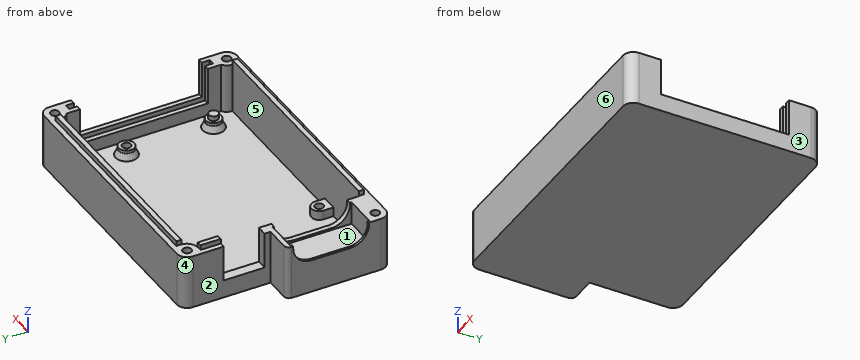
```python
from build123d import *

# Parameters (mm, degrees)
PAD_DEPTH       = 1.5
PAD001_DEPTH    = 15.9
SKETCH003_R     = 2.5
PAD002_DEPTH    = 3
SKETCH004_R     = 1.5
PAD003_DEPTH    = 1.6
SKETCH005_W     = 70.1
SKETCH005_H     = 1.6
SKETCH005_W_2   = 1.6
SKETCH005_H_2   = 11.9
SKETCH005_W_3   = 73.4
PAD004_DEPTH    = 1.6
SKETCH007_W     = 1.9
SKETCH007_H     = 46.1
POCKET001_DEPTH = 14.35
SKETCH008_W     = 5.6
SKETCH008_H     = 41.02
POCKET002_DEPTH = 11.81
SKETCH009_W     = 4.8
SKETCH009_H     = 13.1
POCKET003_DEPTH = 13.2
SKETCH010_R     = 1.4
POCKET004_DEPTH = 15.9
POCKET_DEPTH    = 6.7
SKETCH014_W     = 10.3
SKETCH014_H     = 25.3
POCKET006_DEPTH = 0.65
SKETCH023_R     = 1.4
POCKET014_DEPTH = 4
CHAMFER_SIZE2   = 2
CHAMFER_SIZE    = 1
FILLET_R        = 3.3
FILLET001_R     = 1.6
FILLET002_R     = 6


with BuildPart() as part:
    # Sketch → Pad (new body)
    with BuildSketch(Plane.XY):
        Polygon((13.3, 49.3), (13.3, 77.5), (96.8, 77.5), (96.8, 15.8), (3.9, 15.8), (3.9, 49.3), align=None)
    extrude(amount=PAD_DEPTH)

    # Sketch001 (on Face8 of Pad) → Pad001 (join)
    with BuildSketch(Plane.XY.offset(1.5)):
        Polygon((96.8, 77.5), (13.3, 77.5), (13.3, 49.3), (3.9, 49.3), (3.9, 15.8), (96.8, 15.8), align=None)
        with BuildLine():
            Line((16.6, 70.9), (16.6, 19.1))
            Line((16.6, 19.1), (90.2, 19.1))
            ThreePointArc((91.7, 21.865863), (90.599138, 20.673213), (90.2, 19.1))
            Line((91.7, 21.865863), (91.7, 71.434137))
            ThreePointArc((90.2, 74.2), (90.599138, 72.626787), (91.7, 71.434137))
            Line((90.2, 74.2), (19.9, 74.2))
            ThreePointArc((16.6, 70.9), (18.933452, 71.866548), (19.9, 74.2))
        make_face(mode=Mode.SUBTRACT)
    extrude(amount=PAD001_DEPTH)

    # Sketch003 (on Face9 of Pad001) → Pad002 (join)
    with BuildSketch(Plane.XY.offset(1.5)):
        with Locations((86, 55.35)):
            Circle(SKETCH003_R)
        with Locations((86, 27.45)):
            Circle(SKETCH003_R)
        with BuildLine():
            ThreePointArc((36.4, 22.35), (33.9, 24.85), (31.4, 22.35))
            Line((31.4, 22.35), (31.4, 18))
            Line((36.4, 18), (31.4, 18))
            Line((36.4, 22.35), (36.4, 18))
        make_face()
        with BuildLine():
            ThreePointArc((32.95, 70.55), (35.2, 68.3), (37.45, 70.55))
            Line((37.45, 70.55), (37.45, 75.55))
            Line((32.95, 75.55), (37.45, 75.55))
            Line((32.95, 70.55), (32.95, 75.55))
        make_face()
    extrude(amount=PAD002_DEPTH)

    # Sketch004 (on Face28 of Pad002) → Pad003 (join)
    with BuildSketch(Plane.XY.offset(4.5)):
        with Locations((35.2, 70.55)):
            Circle(SKETCH004_R)
        with Locations((86, 27.45)):
            Circle(SKETCH004_R)
    extrude(amount=PAD003_DEPTH)

    # Sketch005 (on Face1 of Pad003) → Pad004 (join)
    with BuildSketch(Plane.XY.offset(17.4)):
        with Locations((55.05, 75)):
            Rectangle(SKETCH005_W, SKETCH005_H)
        with Locations((15.8, 64.85)):
            Rectangle(SKETCH005_W_2, SKETCH005_H_2)
        with Locations((53.4, 18.3)):
            Rectangle(SKETCH005_W_3, SKETCH005_H)
    extrude(amount=PAD004_DEPTH)

    # Sketch007 (on Face1 of Pad004) → Pocket001 (cut)
    with BuildSketch(Plane.XY.offset(17.4)):
        with Locations((94.25, 46.65)):
            Rectangle(SKETCH007_W, SKETCH007_H)
    extrude(amount=-POCKET001_DEPTH, mode=Mode.SUBTRACT)

    # Sketch008 (on Face1 of Pocket001) → Pocket002 (cut)
    with BuildSketch(Plane.XY.offset(17.4)):
        with Locations((94.25, 46.65)):
            Rectangle(SKETCH008_W, SKETCH008_H)
    extrude(amount=-POCKET002_DEPTH, mode=Mode.SUBTRACT)

    # Sketch009 (on Face41 of Pocket002) → Pocket003 (cut)
    with BuildSketch(Plane.XY.offset(19)):
        with Locations((14.6, 57.75)):
            Rectangle(SKETCH009_W, SKETCH009_H)
    extrude(amount=-POCKET003_DEPTH, mode=Mode.SUBTRACT)

    # Sketch010 (on Face1 of Pocket003) → Pocket004 (cut)
    with BuildSketch(Plane.XY.offset(17.4)):
        with Locations((16.6, 74.2)):
            Circle(SKETCH010_R)
        with Locations((93.5, 74.2)):
            Circle(SKETCH010_R)
        with Locations((93.5, 19.1)):
            Circle(SKETCH010_R)
        with Locations((7.2, 19.1)):
            Circle(SKETCH010_R)
    extrude(amount=-POCKET004_DEPTH, mode=Mode.SUBTRACT)

    # Sketch002 (on Face1 of Pad001) → Pocket (cut)
    with BuildSketch(Plane.XY.offset(17.4)):
        Polygon((4.7, 22.4), (15, 22.4), (15, 22.9), (18.2, 22.9), (18.2, 47.2), (15, 47.2), (15, 47.7), (4.7, 47.7), (4.7, 47.2), (1.5, 47.2), (1.5, 22.9), (4.7, 22.9), align=None)
    extrude(amount=-POCKET_DEPTH, mode=Mode.SUBTRACT)

    # Sketch014 (on Face41 of Pocket) → Pocket006 (cut)
    with BuildSketch(Plane.XY.offset(10.7)):
        with Locations((9.85, 35.05)):
            Rectangle(SKETCH014_W, SKETCH014_H)
    extrude(amount=-POCKET006_DEPTH, mode=Mode.SUBTRACT)

    # Sketch023 (on Face70 of Pocket006) → Pocket014 (cut)
    with BuildSketch(Plane.XY.offset(4.5)):
        with Locations((33.9, 22.35)):
            Circle(SKETCH023_R)
        with Locations((86, 55.35)):
            Circle(SKETCH023_R)
    extrude(amount=-POCKET014_DEPTH, mode=Mode.SUBTRACT)

    # Chamfer
    chamfer_edges = [part.edges().sort_by_distance(p)[0] for p in [
        (83.5, 55.35, 1.5),
        (83.5, 27.45, 1.5),
    ]]
    chamfer_side = part.faces().sort_by_distance((54.108445, 46.65668, 1.5))[0]
    chamfer(chamfer_edges, length=CHAMFER_SIZE, length2=CHAMFER_SIZE2, reference=chamfer_side)

    # Fillet
    fillet_edges = [part.edges().sort_by_distance(p)[0] for p in [
        (13.3, 77.5, 8.7),
        (3.9, 15.8, 8.7),
        (96.8, 77.5, 8.7),
        (96.8, 15.8, 8.7),
    ]]
    fillet(fillet_edges, radius=FILLET_R)

    # Fillet001
    fillet001_edges = [part.edges().sort_by_distance(p)[0] for p in [
        (3.9, 49.3, 8.7),
    ]]
    fillet(fillet001_edges, radius=FILLET001_R)

    # Fillet002
    fillet002_edges = [part.edges().sort_by_distance(p)[0] for p in [
        (15.8, 22.9, 10.7),
        (15.8, 47.2, 10.7),
        (4.3, 47.2, 10.7),
        (4.3, 22.9, 10.7),
    ]]
    fillet(fillet002_edges, radius=FILLET002_R)


solid = part.part
```
Verification items for the finished model (mm, model axes). Face numbers are marked on the shaded views. A direction names the side the tool comes from. Give positions to 0.01 mm unless a question says otherwise; leave off trailing zeros. Order: outer loops, then holes, each group sorted by start corner. A loop starts at its lowest first (then second) coordinate and runs counter-clockwise, first axis right, second up. Notation, with made-up numbers: (68.25, 59) - (120.25, 59) arc R22 ccw to (120.25, 78) - close; hole circle Ø8 at (-1.75, 70.25). An arc over 180 degrees is marked (long way). Answer as CSV lines item,"result". Start each with the question number.
Item 1: Section check C-C, the plane z = 12.75. State how many separate pieces and enclosed holes the cut face has, plus the area to 3 significant figures.
Item 2: Gauge pin test, flat ends, axial feed: pin 1 (0.5 mm diameter, centred on x = 15.5, z = 18.5, fed in from +Y); pin 2 (8 mm diameter, centred on x = 29, y = 67, fed in from +Z); pin 3 (0.6 mm diameter, centred on x = 15.5, z = 17, fed in from +Y). Record the tip position at first contact, or that the pin passes through.
Item 3: Section check A-A, the plane y = 66. Record the boundary of the cut face in (x, z).
Item 4: Section check D-D, the plane y = 32.5. Record the boundary of the cut face in (x, z), plus the area to 3 significant figures.
Item 5: Access from +Z, -Z, +X, -X, +Y, -Y to the whole of each face (thin tool, end or side, straight path). Record for the marked faces 1, 2 and 3.
Item 6: Material ranges on L1, parallel to Y at x = 93.5, z = 7.5; L2, parallel to Y at x = 27, z = 15.5; L3, parallel to X at y = 46.5, z = 5.25, recorded low to high.
Item 7: Section check B-B, the plane x = 38.5. Record the boundary of the cut face in (y, z), plus the area to 3 significant figures.
Item 8: Mould release check, pull along Y, two halves, no side actions. Record for the marked faces 4, 5 and 6: released by +Y, released by -Y, zero draft, split by the parting line, or undercut.
Filled in:
1,separate pieces,"3"
1,enclosed holes,"4"
1,area,"735 mm^2"
2,pin 1,"y = 70.8"
2,pin 2,"z = 1.5"
2,pin 3,"y = 77.4"
3,outline,"(13.3, 0) - (96.8, 0) - (96.8, 5.59) - (95.2, 5.59) - (95.2, 3.05) - (93.3, 3.05) - (93.3, 5.59) - (91.7, 5.59) - (91.7, 1.5) - (16.6, 1.5) - (16.6, 19) - (15, 19) - (15, 17.4) - (13.3, 17.4) - close"
4,outline,"(3.9, 0) - (96.8, 0) - (96.8, 5.59) - (95.2, 5.59) - (95.2, 3.05) - (93.3, 3.05) - (93.3, 5.59) - (91.7, 5.59) - (91.7, 1.5) - (16.6, 1.5) - (16.6, 10.7) - (15, 10.7) - (15, 10.05) - (4.7, 10.05) - (4.7, 10.7) - (3.9, 10.7) - close"
4,area,"266 mm^2"
5,face 1,"+Z"
5,face 2,"+Z, -Z, -X, +Y"
5,face 3,"+Z, -Z, +X, +Y, -Y"
6,L1,"15.8 to 17.7, 20.5 to 23.6, 69.7 to 72.8, 75.6 to 77.5"
6,L2,"15.8 to 19.1, 74.2 to 77.5"
6,L3,"3.9 to 16.6, 91.7 to 93.3, 95.2 to 96.8"
7,outline,"(15.8, 0) - (77.5, 0) - (77.5, 17.4) - (75.8, 17.4) - (75.8, 19) - (74.2, 19) - (74.2, 1.5) - (19.1, 1.5) - (19.1, 19) - (17.5, 19) - (17.5, 17.4) - (15.8, 17.4) - close"
7,area,"203 mm^2"
8,face 4,"released by +Y"
8,face 5,"undercut"
8,face 6,"released by -Y"
